Check sheet for the modelled part. Datum: model origin and axes. Units: mm. A direction names the side the tool comes from. Round coordinates to 2 decimals unless told otherwise and drop trailing zeros. Order: outer loops, then holes, each group sorted by start corner. A loop starts at its lowest first (then second) coordinate and runs counter-clockwise, first axis right, second up.
(1) Sectioned sample at C-C, the plane z = 1.4. Count the separate pieces of the cut face and the enclosed holes in it, and give its area (3 significant figures).
(2) Sectioned sample at B-B, the plane y = 25.5. Enter the section's corners in (x, z).
(3) Sectioned sample at A-A, the plane x = -73. Enter the section's corners in (y, z).
(4) Depth check by flat-ended pin: pin 1 (3.5 mm diameter, centred on x = -84.8, y = 15.5, fed in from +Z). Enter the tip coordinate at first touch or a pass-through.
(5) Sectioned sample at D-D, the plane x = -84.8. Enter the section's corners in (y, z), and give its area (3 significant figures).
(6) Thickness scan on probe 1 along X at (y, z) = (13.5, 1.45); probe 2 along X at (y, z) = (28, 0.65); probe 3 along X at (y, z) = (36, 0.3). Record the ranges inside material, lowest first.
(7) Mould release check, pull along Y, two halves, no side actions. Record for faces 3 (the flat face through (-23, 36, 1)), 4 (the flat face through (-50.05, 5, 1)), 5 (the flat face through (0, 30.5, 1)): released by +Y, released by -Y, zero draft, split by the parting line, or undercut.
(8) Tool access check on faces 1 (the flat face through (-35, 0, 1)), 2 (the flat face through (-15, 10, 1)). Record the directions out of +Z, -Z, +X, -X, +Y, -Y that give a thin tool (end or side, any length) a straight path to the whole face; none if there is none.
```python
from build123d import *

# Parameters (mm, degrees)
ESBO_O1_W                = 20
ESBO_O1_H                = 3
ESBO_O1_R                = 1.6
ESBO_O1_W_2              = 42
ESBO_O1_H_2              = 21
ESBO_O1_W_3              = 3
ESBO_O1_H_3              = 10
ESBO_O1_R_2              = 2.6
RESSALTO_EXTRUS_O1_DEPTH = 3


with BuildPart() as part:
    # Esboço1 → Ressalto-extrusão1 (new body)
    with BuildSketch(Plane.XY):
        Polygon((-23, 0), (23, 0), (23, 30.5), (-23, 30.5), (-23, 41), (-91.05, 41), (-91.05, 0), align=None)
        with Locations((-60.05, 5)):
            Rectangle(ESBO_O1_W, ESBO_O1_H, mode=Mode.SUBTRACT)
        with Locations((-84.8, 15.5)):
            Circle(ESBO_O1_R, mode=Mode.SUBTRACT)
        with Locations((-60.05, 20.5)):
            Rectangle(ESBO_O1_W_2, ESBO_O1_H_2, mode=Mode.SUBTRACT)
        with Locations((-35.3, 15.5)):
            Circle(ESBO_O1_R, mode=Mode.SUBTRACT)
        with Locations((-16.5, 10)):
            Rectangle(ESBO_O1_W_3, ESBO_O1_H_3, mode=Mode.SUBTRACT)
        with Locations((16.5, 10)):
            Rectangle(ESBO_O1_W_3, ESBO_O1_H_3, mode=Mode.SUBTRACT)
        with Locations((0, 20.5)):
            Circle(ESBO_O1_R_2, mode=Mode.SUBTRACT)
        with Locations((-84.8, 25.5)):
            Circle(ESBO_O1_R, mode=Mode.SUBTRACT)
        with Locations((-35.3, 25.5)):
            Circle(ESBO_O1_R, mode=Mode.SUBTRACT)
        with Locations((-60.05, 36)):
            Rectangle(ESBO_O1_W, ESBO_O1_H, mode=Mode.SUBTRACT)
    extrude(amount=RESSALTO_EXTRUS_O1_DEPTH)


solid = part.part
```
Derived:
1. separate pieces: 1
1. enclosed holes: 10
1. area: 3,080 mm2
2. outline: (-91.05, 0) - (-86.4, 0) - (-86.4, 3) - (-91.05, 3) - close; (-83.2, 0) - (-81.05, 0) - (-81.05, 3) - (-83.2, 3) - close; (-39.05, 0) - (-36.9, 0) - (-36.9, 3) - (-39.05, 3) - close; (-33.7, 0) - (23, 0) - (23, 3) - (-33.7, 3) - close
3. outline: (0, 0) - (10, 0) - (10, 3) - (0, 3) - close; (31, 0) - (41, 0) - (41, 3) - (31, 3) - close
4. pin 1: stops at z = 3
5. outline: (0, 0) - (13.9, 0) - (13.9, 3) - (0, 3) - close; (17.1, 0) - (23.9, 0) - (23.9, 3) - (17.1, 3) - close; (27.1, 0) - (41, 0) - (41, 3) - (27.1, 3) - close
5. area: 104 mm2
6. probe 1: x = -91.05 to -81.05, -39.05 to -18, -15 to 15, 18 to 23
6. probe 2: x = -91.05 to -81.05, -39.05 to 23
6. probe 3: x = -91.05 to -70.05, -50.05 to -23
7. face 3: zero draft
7. face 4: undercut
7. face 5: released by +Y
8. face 1: +Z, -Z, +X, -X, -Y
8. face 2: +Z, -Z
